Check sheet for the drawn part. Datum: minimum x, y, z corner. Units: mm. A direction names the side the tool comes from. Round coordinates to 2 decimals unless told otherwise and drop trailing zeros. Write each loop counter-clockwise with the first axis right and the second up, starting at its lowest first coordinate (ties: lowest second). Pieces come first, ordered by that corner, then holes. Notation, with made-up numbers: M 22.5,51.5 L 51.5,51.5 A15 ccw 51.5,66.5 Z; hole C 15.25,-27 d8. An arc over 180 degrees is marked long. One line per item, written item: value. Start each with the question number.
Item 1: Section check B-B, the plane z = 101.6. Record the cut outline in (x, y).
Item 2: Gauge pin test, flat end, axial feed: pin 1 (1.5 mm diameter, centred on x = 55, z = 27, fed in from +Y). Record the tip position at first contact, or that the pin passes through.
Item 3: Section check C-C, the plane y = 40. Record the cut outline in (x, z), then the cut area to 3 significant figures.
Item 4: Draft check along X on the marked faces 1, 2, 3 and 4. Enter one of: +X half, -X half, draft (parallel to the pull), parting line (faces both ways), or undercut.
Item 5: Thickness scan on probe 1 along X at (y, z) = (3.75, 101.6); probe 2 along X at (y, z) = (33, 96). Record the ranges inside material, lowest first. Write a range as from..to.
Item 6: Tool access check on the marked faces 5 and 6. Record the directions out of +Z, -Z, +X, -X, +Y, -Y that give a thin tool (end or side, any length) a straight path to the whole face; none if there is none.
Item 7: Section check A-A, the plane x = 101.6. Record the cut outline in (y, z).
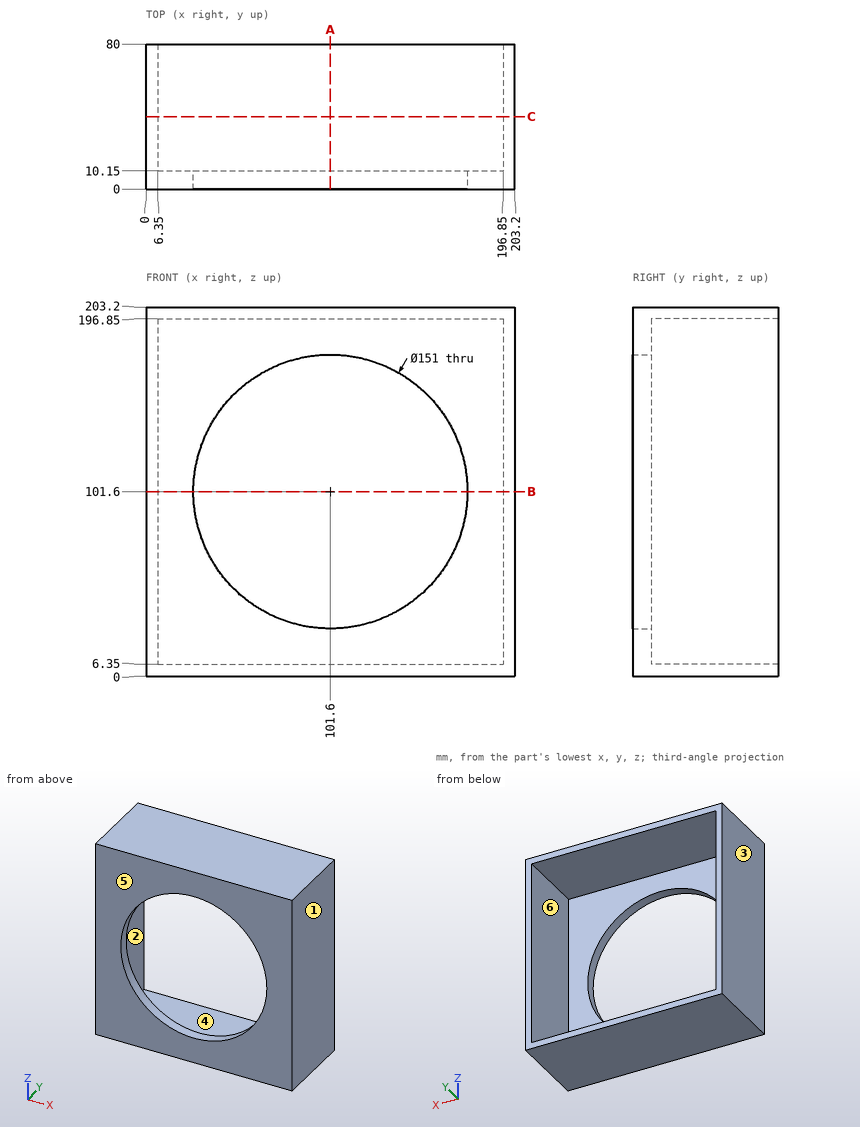
Response values:
1. outline: M 0,0 L 26.1,0 L 26.1,10.15 L 6.35,10.15 L 6.35,80 L 0,80 Z; M 177.1,0 L 203.2,0 L 203.2,80 L 196.85,80 L 196.85,10.15 L 177.1,10.15 Z
2. pin 1: stops at y = 10.15
3. outline: M 0,0 L 203.2,0 L 203.2,203.2 L 0,203.2 Z; hole M 6.35,6.35 L 196.85,6.35 L 196.85,196.85 L 6.35,196.85 Z
3. area: 5,000 mm2
4. face 1: +X half
4. face 2: undercut
4. face 3: -X half
4. face 4: undercut
5. probe 1: x = 0..26.1, 177.1..203.2
5. probe 2: x = 0..6.35, 196.85..203.2
6. face 5: +Z, -Z, +X, -X, -Y
6. face 6: +Y
7. outline: M 0,0 L 80,0 L 80,6.35 L 10.15,6.35 L 10.15,26.1 L 0,26.1 Z; M 0,177.1 L 10.15,177.1 L 10.15,196.85 L 80,196.85 L 80,203.2 L 0,203.2 Z
